Geometry check sheet. Reference: the model listing, model coordinates, mm. A direction names the side the tool comes from. Round coordinates to 2 decimals unless told otherwise and drop trailing zeros. Order: outer loops, then holes, each group sorted by start corner. A loop starts at its lowest first (then second) coordinate and runs counter-clockwise, first axis right, second up. Notation, with made-up numbers: (35.5, -1) - (77.5, -1) arc R28 ccw to (77.5, 21) - close; hole circle Ø6 at (-21.5, 4). An arc over 180 degrees is marked (long way). Use a Markdown table: item, result. Add a question column.
(1) Thickness scan on line 1 along Y through (x, z) = (-8, -0.25); line 2 along Y through (x, z) = (-1.75, 2.5); line 3 along Z through (x, y) = (2.5, 32.5). Record the ranges inside material, lowest first. Write a range as [from, to].
(2) Section check B-B on y = 12. Record the boundary of the cut face in (x, z), then the cut area to 3 significant figures.
(3) Section check A-A on x = 0. Record the boundary of the cut face in (y, z).
(4) Access from +Z, -Z, +X, -X, +Y, -Y to the whole of each face (thin tool, end or side, straight path). Record for faces 1 (the face through (-4.515, 0.271, -7.885)), 2 (the face through (0.45, 46.96, 1.43)).
(5) Mould release check, pull along Z, two halves, no side actions. Record for faces 3 (the face through (0, 49.5, 0)), 4 (the face through (-4.57, 0.27, 7.85)), 5 (the face through (9.086, 0.271, 0.032)), 6 (the face through (4.57, 0.27, -7.85)): released by +Z, released by -Z, zero draft, split by the parting line, or undercut.
(6) Gauge pin test, flat ends, axial feed: P1, Ø1, axis at x = 6.5, z = 6.5, coming from the -Y side; P2, Ø3, axis at y = 14, z = 3, coming from the +X side; P3, Ø5, axis at x = 1.5, z = -5, coming from the +Y side; P4, Ø1, axis at x = 1, y = 10.5, coming from the -Z side. Record the tip position at first contact, or that the pin passes through.
(7) Section check C-C on x = 7. Record the boundary of the cut face in (y, z).
```python
from build123d import *

# Parameters (mm, degrees)
P_IDAT_VYSUNUT_M1_DEPTH = 4.5
SKICA2_R                = 6
P_IDAT_VYSUNUT_M2_DEPTH = 40
SKICA3_R                = 1.5
P_IDAT_VYSUNUT_M3_DEPTH = 5
ZKOSEN_1_SIZE           = 0.5


with BuildPart() as part:
    # Skica1 → Přidat vysunutím1 (new body)
    with BuildSketch(Plane(origin=(0, 0, 0), x_dir=(1, 0, 0), z_dir=(0, 1, 0))):
        Polygon((9.814954576, 0), (4.907477288, 8.5), (-4.907477288, 8.5), (-9.814954576, 0), (-4.907477288, -8.5), (4.907477288, -8.5), align=None)
    extrude(amount=P_IDAT_VYSUNUT_M1_DEPTH)

    # Skica2 → Přidat vysunutím2 (add)
    with BuildSketch(Plane(origin=(0, 4.5, 0), x_dir=(1, 0, 0), z_dir=(0, 1, 0))):
        with Locations(Location((0, 0, 0), (0, 0, 270))):
            Circle(SKICA2_R)
    extrude(amount=P_IDAT_VYSUNUT_M2_DEPTH)

    # Skica3 → Přidat vysunutím3 (add)
    with BuildSketch(Plane(origin=(0, 44.5, 0), x_dir=(1, 0, 0), z_dir=(0, 1, 0))):
        with Locations(Location((0, 0, 0), (0, 0, 270))):
            Circle(SKICA3_R)
    extrude(amount=P_IDAT_VYSUNUT_M3_DEPTH)

    # Skica4 → Odebrat rotací1 (revolve, cut)
    with BuildSketch(Plane.XY):
        Polygon((-9.814954576, 0.999848989), (-8.815105588, 0), (-9.814954576, 0), align=None)
    revolve(axis=Axis((0, 0, 0), (0, 1, 0)), mode=Mode.SUBTRACT)

    # Zkosení1
    zkosen_1_edges = [part.edges().sort_by_distance(p)[0] for p in [
        (0, 44.5, -6),
    ]]
    chamfer(zkosen_1_edges, length=ZKOSEN_1_SIZE)


solid = part.part
```
Check sheet entries:
| question | item | result |
|---|---|---|
| 1 | line 1 | y = [0, 4.5] |
| 1 | line 2 | y = [0, 44.5] |
| 1 | line 3 | z = [-5.45, 5.45] |
| 2 | outline | circle Ø12 at (0, 0) |
| 2 | area | 113 mm2 |
| 3 | outline | (0, -8.5) - (4.5, -8.5) - (4.5, -6) - (44, -6) - (44.5, -5.5) - (44.5, -1.5) - (49.5, -1.5) - (49.5, 1.5) - (44.5, 1.5) - (44.5, 5.5) - (44, 6) - (4.5, 6) - (4.5, 8.5) - (0, 8.5) - close |
| 4 | face 1 | -Z, -X, -Y |
| 4 | face 2 | +Y |
| 5 | face 3 | zero draft |
| 5 | face 4 | released by +Z |
| 5 | face 5 | split by the parting line |
| 5 | face 6 | released by -Z |
| 6 | P1 | stops at y = 0 |
| 6 | P2 | stops at x = 5.81 |
| 6 | P3 | stops at y = 44.5 |
| 6 | P4 | stops at z = -5.98 |
| 7 | outline | (0, -4.88) - (4.5, -4.88) - (4.5, 4.88) - (0, 4.88) - close |
